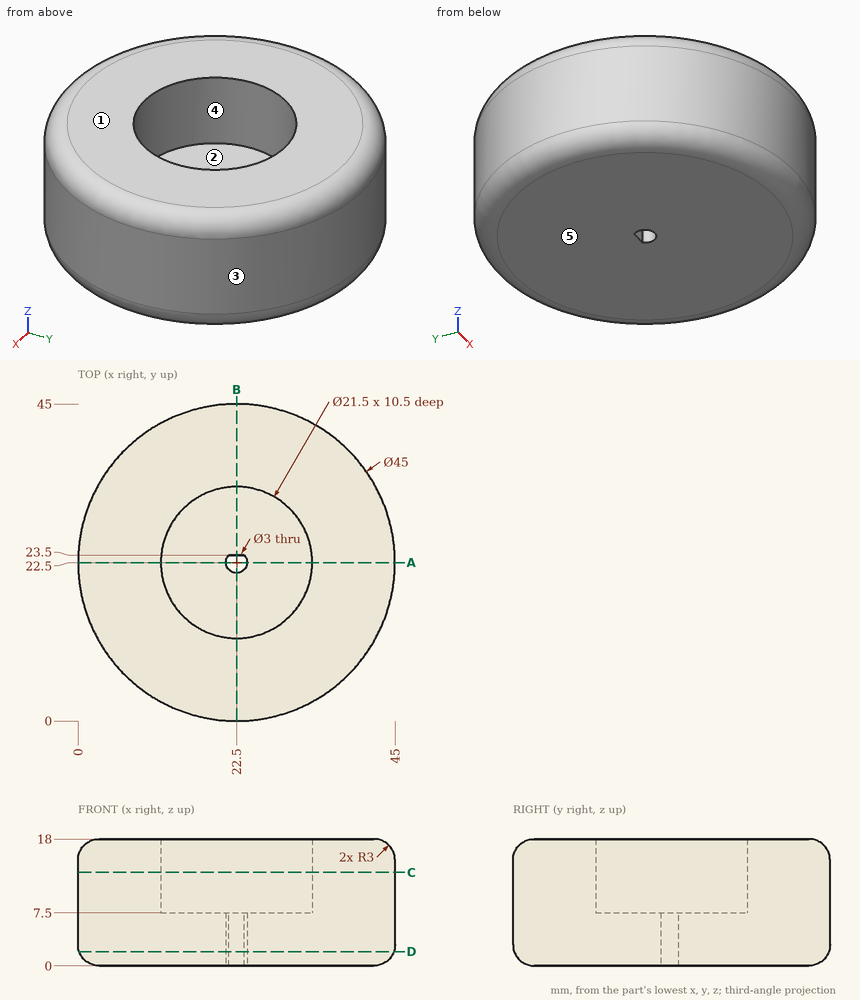
Design review of the part shown in the three views and the two pictorial views. Dimensions are in mm from the part's minimum x, y and z. A direction names the side the tool comes from. Round coordinates to 2 decimals unless told otherwise and drop trailing zeros. Write each loop counter-clockwise with the first axis right and the second up, starting at its lowest first coordinate (ties: lowest second). Pieces come first, ordered by that corner, then holes. Notation, with made-up numbers: M 3.25,-28.5 L 60.25,-28.5 A21 cw 60.25,-6.5 Z; hole C 42,36.25 d3. An arc over 180 degrees is marked long. Use a Markdown table: item, result. Add a question column.
Q1. The part is to be moulded in two halves that separate along Y. For the marked faces 1, 2 and 3, say which applies: pulls with the +Y half, pulls with the -Y half, needs draft (parallel to the pull), parting line crosses it, or undercut.
Q2. We need section D-D, the plane z = 2. State the section outline as (x, y) points, plus the area to 3 significant figures.
Q3. We need section A-A, the plane y = 22.5. State the section outline as (x, z) points.
Q4. To check wall thickness, follow line 1 (Y direction, x = 22.5, z = 10.5); line 2 (Z direction, x = 23, y = 25); line 3 (X direction, y = 27, z = 10.75). State the ranges of each line that lie inside material, in increasing order.
Q5. Insertion check: pin 1 (1.8 mm diameter, centred on x = 22, z = 3, fed in from -Y); pin 2 (8 mm diameter, centred on x = 9, z = 8.5, fed in from -Y); pin 3 (2 mm diameter, centred on y = 13.5, z = 6.5, fed in from -X). Each pin has a flat end and moves straight along its axis. Give the tip position at first contact, or say it passes through.
Q6. Machinability: for the marked faces 4 and 5, which of the approach directions +Z, -Z, +X, -X, +Y, -Y give a long, thin tool a straight path to every point of the face, cutting with its end or side? Answer none if there is none.
Q7. We need section C-C, the plane z = 13.25. State the section outline as (x, y) points, plus the area to 3 significant figures.
Q8. We need section B-B, the plane x = 22.5. State the section outline as (y, z) points, plus the area to 3 significant figures.
Findings below:
| question | item | result |
|---|---|---|
| 1 | face 1 | needs draft |
| 1 | face 2 | undercut |
| 1 | face 3 | parting line crosses it |
| 2 | outline | C 22.5,22.5 d44.66; hole M 21.38,23.5 A1.5 ccw long 23.62,23.5 Z |
| 2 | area | 1,560 mm² |
| 3 | outline | M 0,3 A3 ccw 3,0 L 21,0 L 21,7.5 L 11.75,7.5 L 11.75,18 L 3,18 A3 ccw 0,15 Z; M 24,0 L 42,0 A3 ccw 45,3 L 45,15 A3 ccw 42,18 L 33.25,18 L 33.25,7.5 L 24,7.5 Z |
| 4 | line 1 | y = 0 to 11.75, 33.25 to 45 |
| 4 | line 2 | z = 0 to 7.5 |
| 4 | line 3 | x = 0.45 to 12.74, 32.26 to 44.55 |
| 5 | pin 1 | stops at y = 0 |
| 5 | pin 2 | stops at y = 2.1 |
| 5 | pin 3 | stops at x = 1.47 |
| 6 | face 4 | +Z |
| 6 | face 5 | -Z, +X, -X, +Y, -Y |
| 7 | outline | C 22.5,22.5 d45; hole C 22.5,22.5 d21.5 |
| 7 | area | 1,230 mm² |
| 8 | outline | M 0,3 A3 ccw 3,0 L 21,0 L 21,7.5 L 11.75,7.5 L 11.75,18 L 3,18 A3 ccw 0,15 Z; M 23.5,0 L 42,0 A3 ccw 45,3 L 45,15 A3 ccw 42,18 L 33.25,18 L 33.25,7.5 L 23.5,7.5 Z |
| 8 | area | 558 mm² |
